Autodesk Inventor part; units mm, degrees
ref_plane "YZ Plane" through (0, 0, 0) normal (1, 0, 0) x (0, 1, 0)
ref_plane "XZ Plane" through (0, 0, 0) normal (0, 1, 0) x (-1, 0, 0)
ref_plane "XY Plane" through (0, 0, 0) normal (0, 0, 1) x (1, 0, 0)
sketch "スケッチ1" plane through (0, 0, 0) normal (0, 0, 1) x (1, 0, 0)
  circle A0 centre (0, 0) radius 7
  circle A1 centre (0, 0) radius 12
  line L0 (-5, 4.899) -> (5, 4.899)
  line L1 (5, 4.899) -> (5, -188.5584)
  line L2 (5, -188.5584) -> (-5, -188.5584)
  line L3 (-5, -188.5584) -> (-5, 4.899)
  circle A2 centre (0, -180) radius 7
  circle A3 centre (0, -180) radius 12
  line L4 (10, -193.5584) -> (10, 9.899)
  line L5 (10, 9.899) -> (-10, 9.899)
  line L6 (-10, 9.899) -> (-10, -193.5584)
  line L7 (-10, -193.5584) -> (10, -193.5584)
  point P0 (5, -10.9087)
  point P1 (-5, -10.9087)
  point P2 (-8, 8.9443)
  point P3 (12, 0)
  point P4 (-5, -169.0913)
  point P5 (5, -169.0913)
  point P6 (0, -188.5584)
  point P7 (10, -173.3668)
  point P8 (10, -6.6332)
  point P9 (-10, -6.6332)
  point P10 (-10, -173.3668)
  dimension "d0" = 14
  dimension "d1" = 24
  dimension "d3" = 10
  dimension "d16" = 14
  dimension "d17" = 24
  dimension "d22" = 180
  dimension "d23" = 5
  dimension "d24" = 0
  dimension "d25" = 5
extrude "押し出し1" add sketch "スケッチ1" along normal blind 8 contours A0 L3 A1 L6 L5 L4 L1 | L1 A1 L3 A0 | L1 A3 L3 A1 | A1 L4 A3 L1 | L3 A3 L6 A1 | L4 A1 | A3 L4 L6 L3 A2 L2 L1 | L1 A2 L3 A3 | A1 L6 | A3 L4 | L6 A3 | L5 A1 | L1 L2 L3 A2
properties part number "legparts_03(seven)" material "ABS プラスチック"
Verification items for the finished model (mm, model axes). A direction names the side the tool comes from. Coordinates: 2 decimals unless noted, no trailing zeros. Loops run counter-clockwise (first coordinate to the right, second up) from the corner with the lowest first, then second, coordinate; pieces in that order, holes last. Notation, with made-up numbers: (-30.5, -9) -> (-17.5, -9) arc R21 ccw to (-17.5, -2) -> close; hole circle Ø1 at (-12.75, -23). An arc over 180 degrees is marked (long way). Write each question's results on one line, items separated by ' | '.
Item 1: Section check B-B, the plane y = 0. Enter the section's corners in (x, z), plus the area to 3 significant figures.
Found:
outline: (-12, 0) -> (-7, 0) -> (-7, 8) -> (-12, 8) -> close; (7, 0) -> (12, 0) -> (12, 8) -> (7, 8) -> close | area: 80.0 mm2
Item 2: Material ranges on L1, parallel to Y at x = 0, z = 3.5; L2, parallel to X at y = 0, z = 6.25; L3, parallel to Y at x = -3.25, z = 5.75, recorded low to high.
Found:
L1: y = -192 to -187, -173 to -7, 7 to 12 | L2: x = -12 to -7, 7 to 12 | L3: y = -191.55 to -186.2, -173.8 to -6.2, 6.2 to 11.55
Item 3: Section check D-D, the plane y = -171. Enter the section's corners in (x, z), plus the area to 3 significant figures.
Found:
outline: (-10, 0) -> (10, 0) -> (10, 8) -> (-10, 8) -> close | area: 160 mm2
Item 4: Tool access check on faces 1 (the face through (-10, -89, 4)), 2 (the face through (6.466, 2.681, 3.944)). Record the directions out of +Z, -Z, +X, -X, +Y, -Y that give a thin tool (end or side, any length) a straight path to the whole face; none if there is none.
Found:
face 1: +Z, -Z, -X | face 2: +Z, -Z
Item 5: Mould release check, pull along Y, two halves, no side actions. Record for faces 3 (the face through (0, -89, 8)), 4 (the face through (10, -91, 4)): +Y half, -Y half, draft (parallel to the pull), parting line (faces both ways), or undercut.
Found:
face 3: draft | face 4: undercut
Item 6: Section check C-C, the plane z = 6. Enter the section's corners in (x, y).
Found:
outline: (-10, -173.37) arc R12 ccw (long way) to (10, -173.37) -> (10, -6.63) arc R12 ccw (long way) to (-10, -6.63) -> close; hole circle Ø14 at (0, -180); hole circle Ø14 at (0, 0)
Item 7: Gauge pin test, flat ends, axial feed: pin 1 (3 mm diameter, centred on y = -69, z = 3.5, fed in from +X); pin 2 (1 mm diameter, centred on x = 6, z = 3.5, fed in from +Y); pin 3 (2 mm diameter, centred on x = 2, z = 6.5, fed in from +Y). Record the tip position at first contact, or that the pin passes through.
Found:
pin 1: stops at x = 10 | pin 2: stops at y = 10.67 | pin 3: stops at y = 11.96
Item 8: Section check A-A, the plane x = 0. Enter the section's corners in (y, z).
Found:
outline: (-192, 0) -> (-187, 0) -> (-187, 8) -> (-192, 8) -> close; (-173, 0) -> (-7, 0) -> (-7, 8) -> (-173, 8) -> close; (7, 0) -> (12, 0) -> (12, 8) -> (7, 8) -> close
